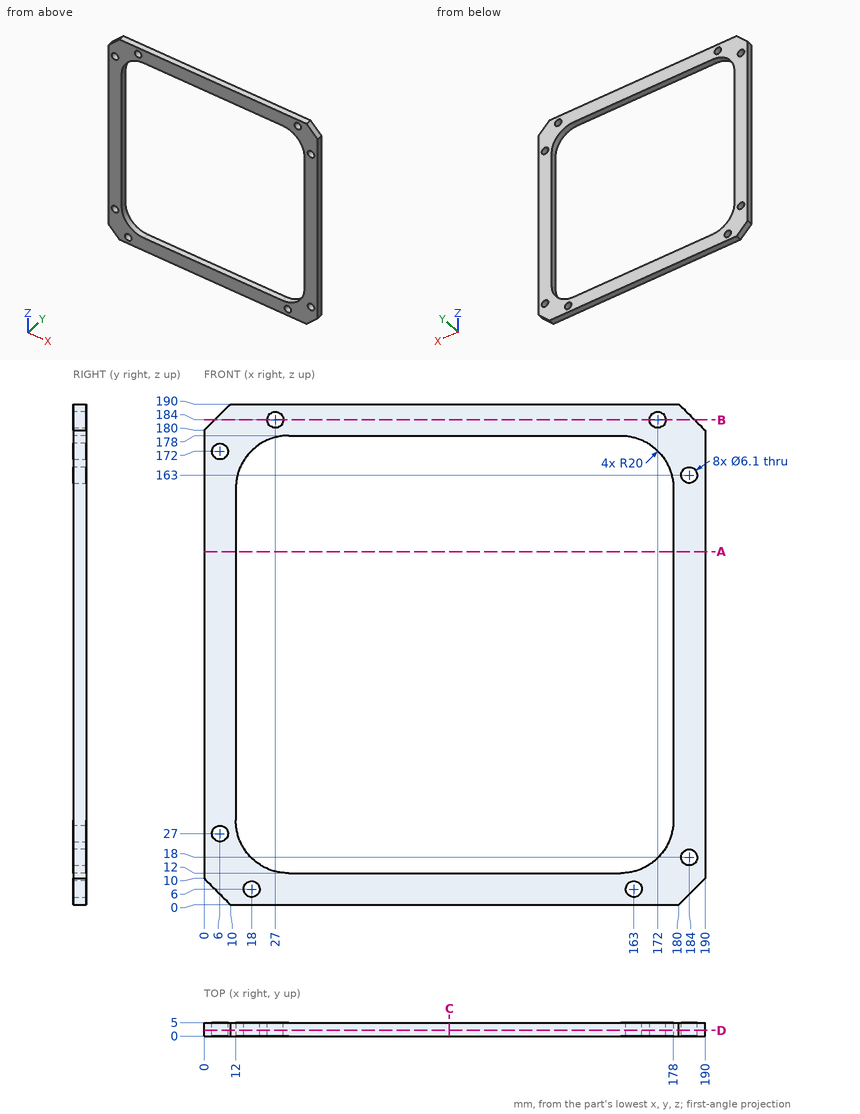
For this review, use the dimensioned drawing (mm, ordinates from the lowest corner) and the shaded views. Round coordinates to 2 decimals unless told otherwise and drop trailing zeros. Order: outer loops, then holes, each group sorted by start corner. A loop starts at its lowest first (then second) coordinate and runs counter-clockwise, first axis right, second up. Notation, with made-up numbers: (33, -9.5) -> (77, -9.5) arc R20 cw to (77, 16.5) -> close; hole circle Ø3 at (72.5, 86.5). An arc over 180 degrees is marked (long way). Write item = value, one per line. Start each with the question number.
Item 1: For line 1 along X through (y, z) = (3.4, 184); line 2 along Z through (x, y) = (163, 1.8); line 3 along X through (y, z) = (2.25, 61.5), list the stretches that pass through material, from the lowest coordinate up.
Item 2: Consider section A-A on z = 134. Write out the cut boundary in (x, y), plus the area to 3 significant figures.
Item 3: Consider section B-B on z = 184. Write out the cut boundary in (x, y), plus the area to 3 significant figures.
Item 4: Consider section C-C on x = 93. Write out the cut boundary in (y, z).
Item 5: Consider section D-D on y = 2.15. Count the separate pieces of the cut face and the enclosed holes in it, plus the area to 3 significant figures.
Conclusion:
q1.line_1 = 4 to 23.95, 30.05 to 168.95, 175.05 to 186
q1.line_2 = 0 to 2.95, 9.05 to 12.64, 177.36 to 190
q1.line_3 = 0 to 12, 178 to 190
q2.outline = (0, 0) -> (12, 0) -> (12, 5) -> (0, 5) -> close; (178, 0) -> (190, 0) -> (190, 5) -> (178, 5) -> close
q2.area = 120 mm2
q3.outline = (4, 0) -> (23.95, 0) -> (23.95, 5) -> (4, 5) -> close; (30.05, 0) -> (168.95, 0) -> (168.95, 5) -> (30.05, 5) -> close; (175.05, 0) -> (186, 0) -> (186, 5) -> (175.05, 5) -> close
q3.area = 849 mm2
q4.outline = (0, 0) -> (5, 0) -> (5, 12) -> (0, 12) -> close; (0, 178) -> (5, 178) -> (5, 190) -> (0, 190) -> close
q5.separate_pieces = 1
q5.enclosed_holes = 9
q5.area = 8,450 mm2
